```python
from build123d import *

# Parameters (mm, degrees)
SKETCH_1_R                   = 1.6
EXTRUDE_1_DEPTH              = 8
EXTRUDE_2_DEPTH              = 15
FILLET_1_R                   = 10
SKETCH_3_R                   = 8.8
CUT_EXTRUDE_1_DEPTH          = 5
SKETCH_4_R                   = 9
SKETCH_4_R_2                 = 1.6000000000000003
EXTRUDE_3_DEPTH              = 2
EXTRUDE_3_DIRECTION_2_REACH  = 64.924
HOLE_WIZARD_M3_1_D           = 3.4
HOLE_WIZARD_M3_1_CBORE_D     = 7
HOLE_WIZARD_M3_1_CBORE_DEPTH = 2.4
HOLE_WIZARD_M3_1_2_D         = 3.4


with BuildPart() as part:
    # 스케치1 → 보스-돌출1 (new body)
    with BuildSketch(Plane.XY):
        with BuildLine():
            Line((-12.16427952654043, 4.378638787940105), (-20.000000000000004, 25))
            Line((-20.000000000000004, 25), (-10.000000000000002, 40.33333333333329))
            Line((-10.000000000000002, 40.33333333333329), (-10.000000000000005, 59.5))
            Line((-10.000000000000005, 59.5), (-5.000000000000006, 59.5))
            Line((-5.000000000000006, 59.5), (-5.000000000000006, 39.5))
            Line((-5.000000000000006, 39.5), (-14.782608695652206, 24.5))
            Line((-14.782608695652206, 24.5), (-3.493383141466383, 9.687944683099722))
            ThreePointArc((-3.493383141466383, 9.687944683099722), (-0.9090438204077795, 7.9117774771707445), (1.988107412927463, 6.7117381440773505))
            ThreePointArc((1.988107412927463, 6.7117381440773505), (5.440021730198806, -4.405242737348851), (-6.151719788633741, -3.3401113218172886))
            ThreePointArc((-6.151719788633741, -3.3401113218172886), (-7.393946440543873, -1.418082905068042), (-8.914100921678212, 0.29260427936827865))
            ThreePointArc((-8.914100921678212, 0.29260427936827865), (-10.673096649546496, 2.229107553388852), (-12.16427952654043, 4.378638787940105))
        make_face()
        Circle(SKETCH_1_R, mode=Mode.SUBTRACT)
    extrude(amount=EXTRUDE_1_DEPTH)

    # 스케치2 → 보스-돌출2 (add)
    with BuildSketch(Plane.XY.offset(8)):
        Polygon((-14.782608695652206, 24.5), (-18.671865990081887, 27.036472148541108), (-10.000000000000002, 40.33333333333329), (-10.000000000000005, 59.5), (-5.000000000000006, 59.5), (-5.000000000000006, 39.5), align=None)
    extrude(amount=-EXTRUDE_2_DEPTH)

    # 필렛1
    fillet_1_edges = [part.edges().sort_by_distance(p)[0] for p in [
        (-14.782608695652206, 24.5, 4),
        (-20.000000000000004, 25, 4),
    ]]
    fillet(fillet_1_edges, radius=FILLET_1_R)

    # 스케치3 → 컷-돌출1 (cut)
    with BuildSketch(Plane.XY.offset(8)):
        Circle(SKETCH_3_R)
    extrude(amount=-CUT_EXTRUDE_1_DEPTH, mode=Mode.SUBTRACT)

    # 스케치4 → 보스-돌출3 (add)
    with BuildSketch(Plane(origin=(0, 0, 0), x_dir=(-1, 0, 0), z_dir=(0, 0, -1))):
        Circle(SKETCH_4_R)
        Circle(SKETCH_4_R_2, mode=Mode.SUBTRACT)
    extrude(amount=EXTRUDE_3_DEPTH)

    # 보스-돌출3 direction 2: up to this face of the body (flat: up to its plane)
    extrude_3_direction_2_end = Plane(part.part.faces().sort_by_distance((-0.17036429, 7.291732251, 3))[0])
    # 스케치4 → 보스-돌출3 direction 2 (add, up to the picked face)
    with BuildSketch(Plane(origin=(0, 0, 0), x_dir=(-1, 0, 0), z_dir=(0, 0, -1)), mode=Mode.PRIVATE) as extrude_3_direction_2_sk1:
        Circle(SKETCH_4_R)
        Circle(SKETCH_4_R_2, mode=Mode.SUBTRACT)
    extrude_3_direction_2_tool1 = split(extrude(extrude_3_direction_2_sk1.sketch, amount=-EXTRUDE_3_DIRECTION_2_REACH, mode=Mode.PRIVATE), bisect_by=extrude_3_direction_2_end, keep=Keep.BOTH, mode=Mode.PRIVATE)
    add(extrude_3_direction_2_tool1.solids().sort_by(Axis((8.745442, 0, 0), (0, 0, 1)))[0])

    # Hole Wizard M3 _ _ _ _1 (through all)
    with Locations(Plane(origin=(0, 0, -2), x_dir=(-1, 0, 0), z_dir=(0, 0, -1))):
        with Locations((0, 6.35), (6.35, 0), (0, -6.35), (-6.35, 0)):
            CounterBoreHole(HOLE_WIZARD_M3_1_D / 2, HOLE_WIZARD_M3_1_CBORE_D / 2, HOLE_WIZARD_M3_1_CBORE_DEPTH)

    # Hole Wizard M3 _ _1 2 (through all)
    with Locations(Plane.ZY.offset(9.999999999999995)):
        with Locations((0.5, 54.5), (0.5, 44.5)):
            Hole(HOLE_WIZARD_M3_1_2_D / 2)


solid = part.part
```
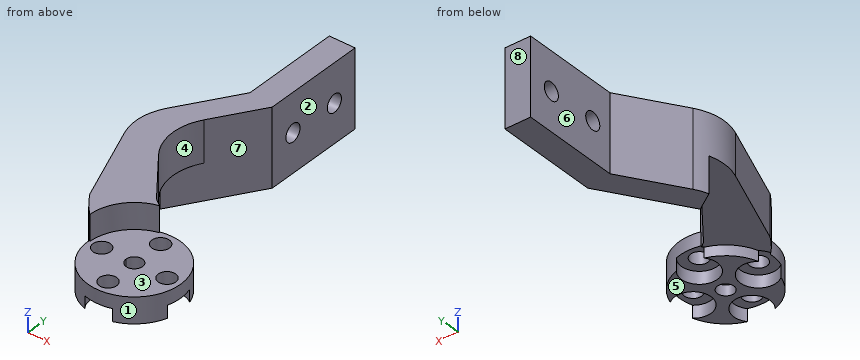
Can you work these out from the model? Positions are in its coordinate system, mm. Face numbers are marked on the shaded views. A direction names the side the tool comes from. Round coordinates to 2 decimals unless told otherwise and drop trailing zeros. Order: outer loops, then holes, each group sorted by start corner. A loop starts at its lowest first (then second) coordinate and runs counter-clockwise, first axis right, second up. Notation, with made-up numbers: (-2.5, 54.25) -> (38.5, 54.25) arc R16 ccw to (38.5, 78.25) -> close; hole circle Ø8 at (29.25, 12.25). An arc over 180 degrees is marked (long way). Return JSON: item names as keys, results as strings. Group by question number.
1. If we section it at C-C, the plane x = 0: Write out the boundary of the cut face in (y, z).
2. If we section it at B-B, the plane x = -7.25: Write out the boundary of the cut face in (y, z).
3. Will these pins go through, and if not, where does the flat tip stop? pin 1 (8 mm diameter, centred on x = 4, y = 3.5, fed in from -Z); pin 2 (5 mm diameter, centred on y = 25, z = 1, fed in from +X); pin 3 (4 mm diameter, centred on x = 0, y = -6.35, fed in from -Z).
4. I need wall thicknesses on line 1 (Y direction, x = 0, z = 1.95); line 2 (X direction, y = -1, z = 1.25); line 3 (Y direction, x = -7.75, z = 0.5). Which ranges of each line are inside material? Lowest first, please. Write a range as [from, to].
5. If we section it at A-A, the plane y = 54.5: Write out the boundary of the cut face in (x, z).
6. We'd pull the mould along Y, two halves only. Please class the marked faces 6, 7 and 8: released by +Y, released by -Y, zero draft, split by the parting line, or undercut.
7. Which directions (+Z, -Z, +X, -X, +Y, -Y) give clear straight access to the entire face, cutting with the end or side of a thin tool? Please do the marked faces 1, 2, 3, 4 and 5.
8. If we section it at D-D, the plane z = -3.5: Write out the boundary of the cut face in (x, y).
Output values:
{
 "1": {"outline": "(-9, 0.4) -> (-8.05, 0.4) -> (-8.05, 3) -> (-9, 3) -> close; (-4.65, 0.4) -> (-2.85, 0.4) -> (-2.85, -2) -> (-1.6, -2) -> (-1.6, 3) -> (-4.65, 3) -> close; (1.6, -2) -> (2.85, -2) -> (2.85, 0.4) -> (4.65, 0.4) -> (4.65, 3) -> (1.6, 3) -> close; (8.05, 0.4) -> (9, 0.4) -> (9, 3) -> (8.05, 3) -> close"},
 "2": {"outline": "(-5.33, -2) -> (-3.38, -2) -> (-3.38, 0.4) -> (-1.44, 0.4) -> (-1.44, 3) -> (-5.33, 3) -> close; (1.44, 0.4) -> (3.38, 0.4) -> (3.38, -2) -> (5.33, -2) -> (5.33, 0) -> (14.62, 0) -> (14.62, 8) -> (4.99, 8) -> (4.99, 3) -> (1.44, 3) -> close; (36.05, -7) -> (59.5, -7) -> (59.5, 8) -> (36.05, 8) -> close; hole circle Ø3.4 at (44.5, 0.5); hole circle Ø3.4 at (54.5, 0.5)"},
 "3": {"pin 1": "z = -2", "pin 2": "x = -12.22", "pin 3": "z = 0.4"},
 "4": {"line 1": "[-9, -8.05], [-4.65, -1.6], [1.6, 4.65], [8.05, 9]", "line 2": "[-8.94, -7.72], [-4.98, -1.25], [1.25, 4.98], [7.72, 8.94]", "line 3": "[-4.58, -0.96], [0.96, 15.27], [35.28, 42.8], [46.2, 52.8], [56.2, 59.5]"},
 "5": {"outline": "(-10, -7) -> (-5, -7) -> (-5, -1.2) -> (-10, -1.2) -> close; (-10, 2.2) -> (-5, 2.2) -> (-5, 8) -> (-10, 8) -> close"},
 "6": {"face 6": "zero draft", "face 7": "undercut", "face 8": "released by +Y"},
 "7": {"face 1": "+Z, -Z", "face 2": "+Z, -Z, +X, +Y", "face 3": "+Z, +X, -Y", "face 4": "+Z, -Z, +X", "face 5": "-Z, +X, -X, -Y"},
 "8": {"outline": "(-18.37, 26.84) -> (-14.78, 24.5) -> (-5, 39.5) -> (-5, 59.5) -> (-10, 59.5) -> (-10, 40.33) -> (-17.22, 29.26) arc R10 ccw to start"}
}
